Geometry: final body of the model. Coordinates: model frame, mm. A direction names the side the tool comes from. Give positions to 0.01 mm unless a question says otherwise; leave off trailing zeros. Write each loop counter-clockwise with the first axis right and the second up, starting at its lowest first coordinate (ties: lowest second). Pieces come first, ordered by that corner, then holes. Notation, with made-up numbers: (84.25, -15) -> (103.25, -15) arc R30 cw to (103.25, 13) -> close; hole circle Ø10 at (77, 69.25). An arc over 180 degrees is marked (long way). Answer in a Markdown table with one row per item. Add a question column.
Item 1: Access query for faces 1 (the flat face through (-109, 21.59, 80)), 2 (the flat face through (-119.63, 11.93, 79.51)), 3 (the flat face through (-102, 0, 88)). Directions: +Z, -Z, +X, -X, +Y, -Y. A direction counts if a zero-diameter tool reaches every point of the face in a straight line with its end or side. Return the directions, or none.
Item 2: Material intervals for probe 1 along Z at (x, y) = (-102, 7.5); probe 2 along Z at (x, y) = (-100.5, 4); probe 3 along X at (y, z) = (9, 89), sorted ascending. Write a range as from..to.
Item 3: Section query A-A on y = 16. Output: boundary loops of the cut face in (x, z), plus the area to 3 significant figures.
Item 4: Section query C-C on z = 93.5. Output: boundary loops of the cut face in (x, y), plus the area to 3 significant figures.
Item 5: First-contact query: P1, Ø7, axis at x = -98, z = 89.5, coming from the +Y side; P2, Ø5, axis at y = 5, z = 81.5, coming from the -X side; P3, Ø3, axis at x = -121.5, z = 74, coming from the -Y side. Flat tips, straight axial feed; report the tip coordinate or a pass-through.
Item 6: Section query B-B on y = 1. Output: boundary loops of the cut face in (x, z).
Item 7: Draft query along Z for faces 4 (the flat face through (-101.47, 11.93, 73.42)), 5 (the flat face through (-103.63, -0.59, 90.51)), 6 (the flat face through (-110.59, 12.2, 84.89)), 7 (the flat face through (-118.499, -0.59, 69.917)). Return one class per face: +Z half, -Z half, draft (parallel to the pull), parting line (faces both ways), or undercut.
```python
from build123d import *
from build123d.topology import SkipClean

# Parameters (mm, degrees)
SKETCH1_R           = 1.5
BOSS_EXTRUDE2_DEPTH = 2.54
BOSS_EXTRUDE3_DEPTH = 19.05
BOSS_EXTRUDE6_DEPTH = 19.05
SKETCH4_R           = 1
CUT_EXTRUDE1_DEPTH  = 158.597711186
FILLET1_R           = 6.35
BOSS_EXTRUDE7_DEPTH = 12.7
SKETCH6_R           = 1.5
CUT_EXTRUDE2_DEPTH  = 159.693396714


with BuildPart() as part:
    # Sketch1 → Boss-Extrude2 (new body)
    with BuildSketch(Plane(origin=(0, 0, 0), x_dir=(1, 0, 0), z_dir=(0, 1, 0))):
        Polygon((-93.521103592, -81.172331094), (-106.459273851, -63.257941504), (-124.37366344, -76.196111763), (-111.435493182, -94.110501353), align=None)
        with Locations(Location((-114.3, -82.55, 0), (0, 0, 270))):
            Circle(SKETCH1_R, mode=Mode.SUBTRACT)
    extrude(amount=BOSS_EXTRUDE2_DEPTH)

    # Sketch2 → Boss-Extrude3 (add)
    with BuildSketch(Plane(origin=(0, 2.54, 0), x_dir=(1, 0, 0), z_dir=(0, 1, 0))):
        Polygon((-106.459273851, -63.257941504), (-124.37366344, -76.196111763), (-111.435493182, -94.110501353), (-93.521103592, -81.172331094), align=None)
        with BuildLine():
            Line((-106.888258276, -65.91764494), (-121.713960005, -76.625096188))
            Line((-121.713960005, -76.625096188), (-118.022197338, -81.736767574))
            ThreePointArc((-118.022197338, -81.736767574), (-117.38868786, -84.78071901), (-114.698271424, -86.339126532))
            Line((-114.698271424, -86.339126532), (-111.006508757, -91.450797917))
            Line((-111.006508757, -91.450797917), (-96.180807028, -80.743346669))
            Line((-96.180807028, -80.743346669), (-106.888258276, -65.91764494))
        make_face(mode=Mode.SUBTRACT)
    extrude(amount=BOSS_EXTRUDE3_DEPTH)

    # Sketch3 → Boss-Extrude6 (add)
    with BuildSketch(Plane(origin=(0, 21.59, 0), x_dir=(1, 0, 0), z_dir=(0, 1, 0))):
        Polygon((-121.713960005, -76.625096188), (-121.188174492, -77.353106899), (-109.675394227, -79.210006941), (-111.53229427, -90.722787207), (-111.006508757, -91.450797917), (-110.278498046, -90.925012404), (-108.421598003, -79.412232139), (-96.908817738, -81.269132182), (-96.180807028, -80.743346669), (-96.706592541, -80.015335958), (-108.219372806, -78.158435915), (-106.362472763, -66.64565565), (-106.888258276, -65.91764494), (-107.616268987, -66.443430453), (-109.473169029, -77.956210718), (-120.985949295, -76.099310675), align=None)
    extrude(amount=-BOSS_EXTRUDE6_DEPTH)

    # Sketch4 → Cut-Extrude1 (cut, through all)
    with BuildSketch(Plane(origin=(6.469085129, 0, 8.957194795), x_dir=(0.8106792283998809, 0, -0.5854905538443587), z_dir=(0.5854905538443586, 0, 0.8106792283998808))):
        with Locations(Location((-134.390249188, 12.7, 0), (0, 0, 90))):
            Circle(SKETCH4_R)
    extrude(amount=-CUT_EXTRUDE1_DEPTH, mode=Mode.SUBTRACT)

    # Fillet1
    fillet1_edges = [part.edges().sort_by_distance(p)[0] for p in [
        (-103.593657892, 2.54, 86.097072293),
        (-114.301109141, 2.54, 71.271370564),
    ]]
    fillet(fillet1_edges, radius=FILLET1_R)

    # Sketch5 → Boss-Extrude7 (add, symmetric)
    with BuildSketch(Plane(origin=(0, 0, 0), x_dir=(-0.8106792283998807, 0, 0.585490553844359), z_dir=(-0.5854905538443589, 0, -0.8106792283998806))):
        Polygon((123.341249188, 0), (145.439249188, 0), (145.439249188, -1.54524269), align=None)
    extrude(amount=BOSS_EXTRUDE7_DEPTH, both=True)

    # Sketch6 → Cut-Extrude2 (cut, through all)
    with SkipClean():  # the faces are left unmerged after this step: merging them gives an invalid solid
        with BuildSketch(Plane(origin=(0, 2.54, 0), x_dir=(1, 0, 0), z_dir=(0, 1, 0))):
            with Locations(Location((-114.3, -82.55, 0), (0, 0, 35.837652954))):
                Circle(SKETCH6_R)
        extrude(amount=-CUT_EXTRUDE2_DEPTH, mode=Mode.SUBTRACT)


solid = part.part
```
Findings below:
| question | item | result |
|---|---|---|
| 1 | face 1 | +Z, -Z, +X, -X, +Y |
| 1 | face 2 | +Y |
| 1 | face 3 | +Z, +X, +Y |
| 2 | probe 1 | z = 69.43..72.69, 79.16..80.45, 84.76..87.3 |
| 2 | probe 2 | z = 71.51..74.76, 79.4..80.69, 81.03..86.21 |
| 2 | probe 3 | x = -115.13..-112.78, -111.25..-109.97, -107.61..-104.36 |
| 3 | outline | (-124.37, 76.2) -> (-106.46, 63.26) -> (-93.52, 81.17) -> (-111.44, 94.11) -> close; hole (-121.19, 77.35) -> (-109.68, 79.21) -> (-111.53, 90.72) -> (-114.7, 86.34) arc R3.81 ccw to (-118.02, 81.74) -> close; hole (-120.99, 76.1) -> (-107.62, 66.44) -> (-109.47, 77.96) -> close; hole (-110.28, 90.93) -> (-108.42, 79.41) -> (-96.91, 81.27) -> close; hole (-108.22, 78.16) -> (-106.36, 66.65) -> (-96.71, 80.02) -> close |
| 3 | area | 211 mm^2 |
| 4 | outline | (-111.88, -1.55) -> (-107.77, -1.31) -> (-107.77, 0) -> (-110.59, 0) -> (-110.59, 21.59) -> (-111.88, 21.59) -> close |
| 4 | area | 33.6 mm^2 |
| 5 | P1 | stops at y = 0 |
| 5 | P2 | stops at x = -122.35 |
| 5 | P3 | stops at y = -1.4 |
| 6 | outline | (-124.37, 76.2) -> (-106.46, 63.26) -> (-93.52, 81.17) -> (-111.44, 94.11) -> close; hole circle Ø3 at (-114.3, 82.55) |
| 7 | face 4 | undercut |
| 7 | face 5 | +Z half |
| 7 | face 6 | undercut |
| 7 | face 7 | -Z half |
